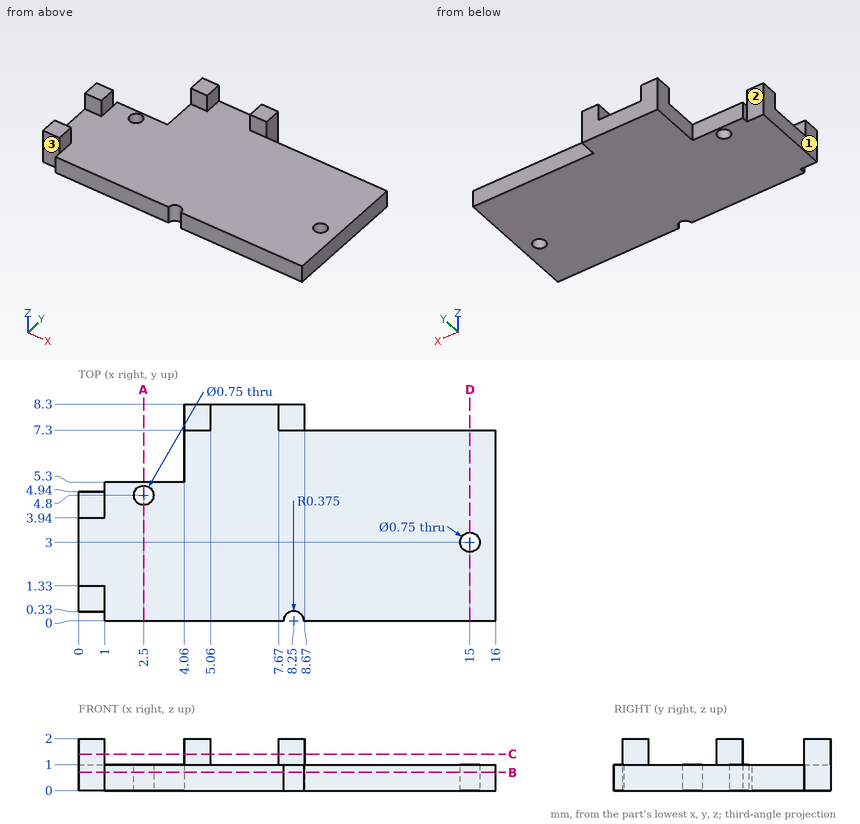
Input: dimensioned drawing with shaded views. Units: mm. Origin: part minimum x, y, z. A direction names the side the tool comes from. Coordinates: 2 decimals unless noted, no trailing zeros. Order: outer loops, then holes, each group sorted by start corner. A loop starts at its lowest first (then second) coordinate and runs counter-clockwise, first axis right, second up. Notation, with made-up numbers: M 80,-11.5 L 121,-11.5 A28 cw 121,15.5 Z; hole C 6.5,26 d3. An arc over 180 degrees is marked long. Write each question's results on one line, items separated by ' | '. Start each with the question number.
Item 1: Cut plane C-C (z = 1.4). Return loops of the section in (x, y), and give its area (3 significant figures).
Item 2: Line query: probe 1 along Y at (x, z) = (15, 0.8) (3 decimals); probe 2 along Z at (x, y) = (14.5, 4); probe 3 along Y at (x, z) = (3, 0.45). Output: solid intervals per line, ascending.
Item 3: First-contact query: pin 1 Ø0.8 at (x, z) = (0.5, 1.5) entering from -Y; pin 2 Ø0.8 at (x, z) = (4.5, 1.5) entering from -Y; pin 3 Ø0.5 at (y, z) = (0.5, 1.5) entering from +X. Flat tips, straight axial feed; report the tip coordinate or a pass-through.
Item 4: Cut plane B-B (z = 0.7). Return loops of the section in (x, y) (3 decimals).
Item 5: Cut plane A-A (x = 2.5). Return loops of the section in (y, z) (3 decimals).
Item 6: Set-up query: the marked faces 1, 2 and 3. Return all of +Z, -Z, +X, -X, +Y, -Y with unobstructed straight access to the full face (end or side cutting, diameter ignored); none if empty.
Item 7: Cut plane D-D (x = 15). Return loops of the section in (y, z) (3 decimals).
Checked values:
1) outline: M 0,0.33 L 1,0.33 L 1,1.33 L 0,1.33 Z; M 0,3.94 L 1,3.94 L 1,4.94 L 0,4.94 Z; M 4.06,7.3 L 5.06,7.3 L 5.06,8.3 L 4.06,8.3 Z; M 7.67,7.3 L 8.67,7.3 L 8.67,8.3 L 7.67,8.3 Z | area: 4.00 mm2
2) probe 1: y = 0 to 2.625, 3.375 to 7.3 | probe 2: z = 0 to 1 | probe 3: y = 0 to 5.3
3) pin 1: stops at y = 0.33 | pin 2: stops at y = 7.3 | pin 3: stops at x = 1
4) outline: M 0,0.33 L 1,0.33 L 1,0 L 7.875,0 A0.375 cw 8.625,0 L 16,0 L 16,7.3 L 8.67,7.3 L 8.67,8.3 L 4.06,8.3 L 4.06,5.3 L 1,5.3 L 1,4.94 L 0,4.94 Z; hole C 2.5,4.8 d0.75; hole C 15,3 d0.75
5) outline: M 0,0 L 4.425,0 L 4.425,1 L 0,1 Z; M 5.175,0 L 5.3,0 L 5.3,1 L 5.175,1 Z
6) face 1: +Z, -Z, -X, +Y, -Y | face 2: +Z, -Z, -X, +Y | face 3: +Z, -Z, -X, -Y
7) outline: M 0,0 L 2.625,0 L 2.625,1 L 0,1 Z; M 3.375,0 L 7.3,0 L 7.3,1 L 3.375,1 Z
